from build123d import *

# Parameters (mm, degrees)
BASEFRAMESKETCH_W           = 15.8
BASEFRAMESKETCH_H           = 3.2
BASEFRAME_DEPTH             = 7.9
STUDSSKETCH_R               = 2.197938665
STUDS_DEPTH                 = 1.6
MAINSTUDSPATTERN_COUNT      = 2
MAINSTUDSPATTERN_PITCH      = 8
MAINSTUDSPATTERN_COUNT_DIR2 = 2
MAINSTUDSPATTERN_PITCH_DIR2 = 8
MAINBASESHELL_T             = -1.2
UNDERCIRCLESKETCH_R         = 3.25
UNDERCIRCLESKETCH_R_2       = 2.4
UNDERCIRCLEEXTRUDE_DEPTH    = 1.8
CUT_EXTRUDE42_DEPTH         = 16.116827041
SKETCH116_R                 = 2.316021132
CUT_EXTRUDE43_DEPTH         = 5
BOSS_EXTRUDE26_START        = -1.2
BOSS_EXTRUDE26_DEPTH        = 1.2


with BuildPart() as part:
    # BaseFrameSketch → BaseFrame (new, symmetric)
    with BuildSketch(Plane.XY):
        with Locations((-4.584729064, 1.6)):
            Rectangle(BASEFRAMESKETCH_W, BASEFRAMESKETCH_H)
    extrude(amount=BASEFRAME_DEPTH, both=True)

    # StudsSketch → Studs (add)
    with BuildSketch(Plane(origin=(0, 3.2, 0), x_dir=(1, 0, 0), z_dir=(0, 1, 0))):
        with Locations((-8.584729064, 4)):
            Circle(STUDSSKETCH_R)
    studs = extrude(amount=STUDS_DEPTH)

    # MainStudsPattern: Studs 2 × 2
    with Locations(*[(i * MAINSTUDSPATTERN_PITCH, 0, j * MAINSTUDSPATTERN_PITCH_DIR2) for i in range(MAINSTUDSPATTERN_COUNT) for j in range(MAINSTUDSPATTERN_COUNT_DIR2) if (i, j) != (0, 0)]):
        add(studs)

    # MainBaseShell
    mainbaseshell_openings = [part.faces().sort_by_distance(p)[0] for p in [
        (-4.584729064, 0, 0),
    ]]
    offset(amount=MAINBASESHELL_T, openings=mainbaseshell_openings, kind=Kind.INTERSECTION)

    # UnderCircleSketch → UnderCircleExtrude (add)
    with BuildSketch(Plane(origin=(0, 2, 0), x_dir=(-1, 0, 0), z_dir=(0, -1, 0))):
        with Locations(Location((4.584729064, 0, 0), (0, 0, 270))):
            Circle(UNDERCIRCLESKETCH_R)
        with Locations(Location((4.584729064, 0, 0), (0, 0, 270))):
            Circle(UNDERCIRCLESKETCH_R_2, mode=Mode.SUBTRACT)
    extrude(amount=UNDERCIRCLEEXTRUDE_DEPTH)

    # Sketch115 → Cut-Extrude42 (cut, through all)
    with BuildSketch(Plane(origin=(0, 3.2, 0), x_dir=(1, 0, 0), z_dir=(0, 1, 0))):
        Polygon((-4.584729064, 7.9), (3.315270936, 7.9), (3.315270936, 0), align=None)
    extrude(amount=-CUT_EXTRUDE42_DEPTH, mode=Mode.SUBTRACT)

    # Sketch116 → Cut-Extrude43 (cut)
    with BuildSketch(Plane(origin=(0, 3.2, 0), x_dir=(1, 0, 0), z_dir=(0, 1, 0))):
        with Locations((-0.622263627, 3.930816352)):
            Circle(SKETCH116_R)
    extrude(amount=CUT_EXTRUDE43_DEPTH, mode=Mode.SUBTRACT)

    # Sketch117 → Boss-Extrude26 (add)
    with BuildSketch(Plane(origin=(0, 3.2, 0), x_dir=(1, 0, 0), z_dir=(0, 1, 0)).offset(BOSS_EXTRUDE26_START)):
        with BuildLine():
            Line((-1.338604614, 4.65387555), (0.069146486, 3.24612445))
            ThreePointArc((0.069146486, 3.24612445), (-1.290378261, 3.294350803), (-1.338604614, 4.65387555))
        make_face()
    extrude(amount=BOSS_EXTRUDE26_DEPTH)


solid = part.part
Input: part model. Units: mm. Frame: model coordinates. A direction names the side the tool comes from. Round coordinates to 2 decimals unless told otherwise and drop trailing zeros. Order: outer loops, then holes, each group sorted by start corner. A loop starts at its lowest first (then second) coordinate and runs counter-clockwise, first axis right, second up. Notation, with made-up numbers: (-19, 74.25) - (-12, 74.25) arc R20 ccw to (-12, 96.25) - close; hole circle Ø5 at (13.5, -18). An arc over 180 degrees is marked (long way). Answer as a JSON object with one key per item and string values. Group by question number.
(1) Reachability of faces 4 (the face through (-1.061, 3.989, 6.146)), 5 (the face through (-0.69, 2.289, -4.005)), 6 (the face through (-9, 4.8, -4)), 7 (the face through (-7, 1, -6.7)), 8 (the face through (-9, 3.6, 4)) from +Z, -Z, +X, -X, +Y, -Y: full face, straight path, thin tool, end or side. Return the list, or none.
(2) Cut plane B-B (x = -8.5). Return loops of the section in (y, z).
(3) Pin query (flat end, axial travel): P1, Ø2, axis at y = 0.5, z = -1.5, coming from the +X side; P2, Ø1, axis at x = -8, z = -4.5, coming from the -Y side; P3, Ø4.5, axis at x = -4.58, z = 0, coming from the +Y side. Return the tip coordinate at first contact, or that it passes through.
(4) Cut plane C-C (z = 6.5). Return loops of the section in (x, y), then the cut area to 3 significant figures.
(5) Draft query along X for faces 1 (the face through (2.115, 1, 3)), 2 (the face through (-9, 4.8, 4)), 3 (the face through (3.315, 2, 4)). Return one class per face: released by +X, released by -X, zero draft, split by the parting line, or undercut.
(6) Material intervals for probe 1 along X at (y, z) = (1.2, 6); probe 2 along X at (y, z) = (2.85, 3.25); probe 3 along X at (y, z) = (2.9, 3.5), sorted ascending. Write a range as from..to.
(7) Cut plane A-A (z = 4). Return loops of the section in (x, y), then the cut area to 3 significant figures.
(8) Cut plane D-D (x = -4). Return loops of the section in (y, z).
Here are the results:
{
 "1": {"face 4": "+Y", "face 5": "-Z, +X, +Y, -Y", "face 6": "+Z, -Z, +X, -X, +Y", "face 7": "+X, -Y", "face 8": "-Y"},
 "2": {"outline": "(0, -7.9) - (3.2, -7.9) - (3.2, -6.2) - (4.8, -6.2) - (4.8, -1.8) - (3.2, -1.8) - (3.2, 1.8) - (4.8, 1.8) - (4.8, 6.2) - (3.2, 6.2) - (3.2, 7.9) - (0, 7.9) - (0, 6.7) - (2, 6.7) - (2, 4.99) - (3.6, 4.99) - (3.6, 3.01) - (2, 3.01) - (2, -3.01) - (3.6, -3.01) - (3.6, -4.99) - (2, -4.99) - (2, -6.7) - (0, -6.7) - close"},
 "3": {"P1": "stops at x = 2.82", "P2": "stops at y = 2", "P3": "stops at y = 3.2"},
 "4": {"outline": "(-12.48, 0) - (-11.28, 0) - (-11.28, 2) - (2.12, 2) - (2.12, 0) - (3.32, 0) - (3.32, 3.2) - (-12.48, 3.2) - close", "area": "23.8 mm^2"},
 "5": {"face 1": "undercut", "face 2": "zero draft", "face 3": "released by +X"},
 "6": {"probe 1": "x = -12.48..-11.28, 2.12..3.32", "probe 2": "x = -12.48..-9.24, -7.93..-1.24, 0.07..3.32", "probe 3": "x = -12.48..-9.45, -7.72..-1.45, 0.28..3.32"},
 "7": {"outline": "(-12.48, 0) - (-11.28, 0) - (-11.28, 2) - (-9.58, 2) - (-9.58, 3.6) - (-7.59, 3.6) - (-7.59, 2) - (-1.58, 2) - (-1.58, 3.6) - (0.41, 3.6) - (0.41, 2) - (2.12, 2) - (2.12, 0) - (3.32, 0) - (3.32, 3.2) - (1.61, 3.2) - (1.61, 4.8) - (-2.78, 4.8) - (-2.78, 3.2) - (-6.39, 3.2) - (-6.39, 4.8) - (-10.78, 4.8) - (-10.78, 3.2) - (-12.48, 3.2) - close", "area": "31.4 mm^2"},
 "8": {"outline": "(0, -7.32) - (3.2, -7.32) - (3.2, 7.9) - (0, 7.9) - (0, 6.7) - (2, 6.7) - (2, 3.2) - (0.2, 3.2) - (0.2, 2.33) - (2, 2.33) - (2, -2.33) - (0.2, -2.33) - (0.2, -3.2) - (2, -3.2) - (2, -6.7) - (0, -6.7) - close"}
}
